Part model, mm, in its own coordinate system. Face numbers are marked on the shaded views. A direction names the side the tool comes from. Round coordinates to 2 decimals unless told otherwise and drop trailing zeros. Loops run counter-clockwise (first coordinate to the right, second up) from the corner with the lowest first, then second, coordinate; pieces in that order, holes last. Notation, with made-up numbers: (-12.5, 67) -> (-1.5, 67) arc R26 cw to (-1.5, 93) -> close; hole circle Ø9 at (-11, -16). An arc over 180 degrees is marked (long way). Answer as a JSON object with one key per item and string values. Group by question number.
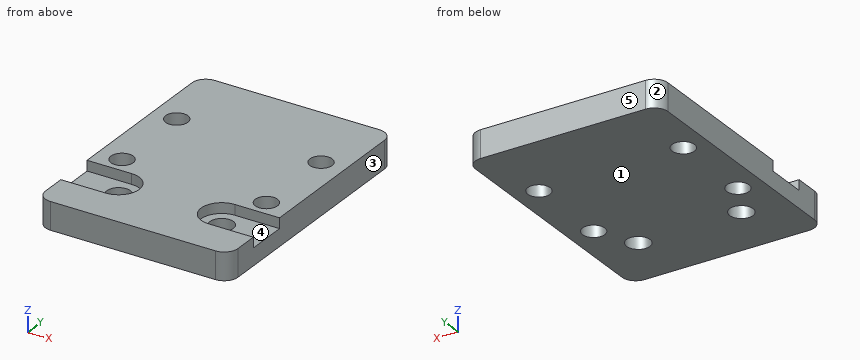
Autodesk Inventor part; units mm, degrees
ref_plane "YZ Plane" through (0, 0, 0) normal (1, 0, 0) x (0, 1, 0)
ref_plane "XZ Plane" through (0, 0, 0) normal (0, 1, 0) x (-1, 0, 0)
ref_plane "XY Plane" through (0, 0, 0) normal (0, 0, 1) x (1, 0, 0)
sketch "Skizze1" plane through (0, 0, 0) normal (0, 0, 1) x (1, 0, 0)
  line L0 (-14, -18.75) -> (14, -18.75)
  line L1 (14, -18.75) -> (14, 18.75)
  line L2 (14, 18.75) -> (-14, 18.75)
  line L3 (-14, 18.75) -> (-14, -18.75)
  line L4 (-14, -18.75) -> (14, 18.75) construction
  line L5 (14, -18.75) -> (-14, 18.75) construction
  circle A0 centre (-10.5, 7.75) radius 1.625
  circle A1 centre (-10.5, -4.75) radius 1.625
  circle A2 centre (10.5, -4.75) radius 1.625
  circle A3 centre (10.5, 7.75) radius 1.625
  line L6 (0, 18.75) -> (0, -18.75) construction
  line L7 (-14, -10.25) -> (14, -10.25) construction
  circle A4 centre (-7.5, -10.25) radius 1.7
  circle A5 centre (7.5, -10.25) radius 1.7
  circle A6 centre (-7.5, -10.25) radius 3
  circle A7 centre (7.5, -10.25) radius 3
  arc A8 (-12, 18.75) -> (-14, 16.75) centre (-12, 16.75) ccw
  arc A9 (14, 16.75) -> (12, 18.75) centre (12, 16.75) ccw
  line L8 (-7.5, -7.25) -> (-14, -7.25)
  line L9 (-7.5, -13.25) -> (-14, -13.25)
  line L10 (-14, -13.25) -> (-14, -7.25)
  line L11 (7.5, -7.25) -> (14, -7.25)
  line L12 (7.5, -13.25) -> (14, -13.25)
  line L13 (14, -13.25) -> (14, -7.25)
  line L14 (-10, -18.75) -> (7, -18.75)
  arc A10 (-14, -16.75) -> (-12, -18.75) centre (-12, -16.75) ccw
  arc A11 (12, -18.75) -> (14, -16.75) centre (12, -16.75) ccw
  point P0 (0, 0)
  point P1 (12.5, -1.6583)
  point P2 (-12.5, -1.6583)
  point P3 (12.5, 1.6583)
  point P4 (-12.5, 1.6583)
  dimension "d0" = 28
  dimension "d1" = 37.5
  dimension "d2" = 3.25
  dimension "d3" = 21
  dimension "d4" = 12.5
  dimension "d6" = 3.4
  dimension "d7" = 15
  dimension "d8" = 6
  dimension "d9" = 2
  dimension "d20" = 11
  dimension "d21" = 29
  dimension "d22" = 8.5
extrude "Extrusion1" add sketch "Skizze1" against normal blind 4 contours A10 L3 L9 A6 L8 A8 L2 A9 L1 L11 A7 L12 A11 L0 | L3 L8 A6 L9 | A6 | L12 A7 L11 L1 | A7
extrude "Extrusion2" cut sketch "Skizze1" against normal blind 1.5 contours L3 L8 A6 L9 | A6 | L12 A7 L11 L1 | A7
properties part number "Camera-Base" material "ABS-Kunststoff"
Item 1: Two-plate mould, pull along X, no slides. Class the marked faces 1, 2 and 3: pulls with the +X half, pulls with the -X half, needs draft (parallel to the pull), parting line crosses it, or undercut.
Item 2: Band-saw the part on D-D, the plane y = -4.75. List the corners of the cut face in (x, z) (3 decimals), plus the area to 3 significant figures.
Item 3: Drill centre lines: line 1 (Y direction, x = 10.5, z = -2.9) (3 decimals); line 2 (Y direction, x = -10.5, z = -1.05) (3 decimals); line 3 (Y direction, x = 7.5, z = -2.55). Where is each one in solid material? Low to high.
Item 4: Drop flat-ended pins along their axis: pin 1 Ø3 at (x, y) = (-10.5, 7.75) entering from -Z; pin 2 Ø5 at (x, y) = (9.5, -10) entering from +Z. Give the stop position or say it passes through.
Item 5: Band-saw the part on A-A, the plane x = 10.5. List the corners of the cut face in (y, z) (3 decimals), plus the area to 3 significant figures.
Item 6: Band-saw the part on C-C, the plane z = -1.95. List the corners of the cut face in (x, y) (3 decimals).
Item 7: Band-saw the part on B-B, the plane y = -10.25. List the corners of the cut face in (x, z), plus the area to 3 significant figures.
Item 8: Which spindle directions (+Z, -Z, +X, -X, +Y, -Y) get a long thin tool onto all of the face, cutting with end or side? Do the marked faces 4 and 5. Say none if no direction does.
Entries:
{
 "1": {"face 1": "needs draft", "face 2": "pulls with the -X half", "face 3": "pulls with the +X half"},
 "2": {"outline": "(-14, -4) -> (-12.125, -4) -> (-12.125, 0) -> (-14, 0) -> close; (-8.875, -4) -> (8.875, -4) -> (8.875, 0) -> (-8.875, 0) -> close; (12.125, -4) -> (14, -4) -> (14, 0) -> (12.125, 0) -> close", "area": "86.0 mm²"},
 "3": {"line 1": "-18.75 to -6.375, -3.125 to 6.125, 9.375 to 18.75", "line 2": "-18.75 to -13.25, -7.25 to -6.375, -3.125 to 6.125, 9.375 to 18.75", "line 3": "-18.75 to -11.95, -8.55 to 18.75"},
 "4": {"pin 1": "through", "pin 2": "z = -1.5"},
 "5": {"outline": "(-18.75, -4) -> (-6.375, -4) -> (-6.375, 0) -> (-7.25, 0) -> (-7.25, -1.5) -> (-13.25, -1.5) -> (-13.25, 0) -> (-18.75, 0) -> close; (-3.125, -4) -> (6.125, -4) -> (6.125, 0) -> (-3.125, 0) -> close; (9.375, -4) -> (18.75, -4) -> (18.75, 0) -> (9.375, 0) -> close", "area": "115 mm²"},
 "6": {"outline": "(-14, -16.75) arc R2 ccw to (-12, -18.75) -> (12, -18.75) arc R2 ccw to (14, -16.75) -> (14, 16.75) arc R2 ccw to (12, 18.75) -> (-12, 18.75) arc R2 ccw to (-14, 16.75) -> close; hole circle Ø3.25 at (-10.5, -4.75); hole circle Ø3.25 at (-10.5, 7.75); hole circle Ø3.4 at (-7.5, -10.25); hole circle Ø3.4 at (7.5, -10.25); hole circle Ø3.25 at (10.5, -4.75); hole circle Ø3.25 at (10.5, 7.75)"},
 "7": {"outline": "(-14, -4) -> (-9.2, -4) -> (-9.2, -1.5) -> (-14, -1.5) -> close; (-5.8, -4) -> (5.8, -4) -> (5.8, -1.5) -> (4.5, -1.5) -> (4.5, 0) -> (-4.5, 0) -> (-4.5, -1.5) -> (-5.8, -1.5) -> close; (9.2, -4) -> (14, -4) -> (14, -1.5) -> (9.2, -1.5) -> close", "area": "66.5 mm²"},
 "8": {"face 4": "+Z, +X", "face 5": "+Z, -Z, +X, -X, +Y"}
}
